```python
from build123d import *

# Parameters (mm, degrees)
BOSS_EXTRUDE2_DEPTH = 6.35
SKETCH5_R           = 1.778
CUT_EXTRUDE1_DEPTH  = 6.35
SKETCH7_W           = 6.35
SKETCH7_H           = 12.7
BOSS_EXTRUDE3_DEPTH = 6.35
SKETCH8_R           = 1.778
CUT_EXTRUDE3_DEPTH  = 6.35
SKETCH9_R           = 1.143
CUT_EXTRUDE4_DEPTH  = 12.7
BOSS_EXTRUDE5_DEPTH = 3.81
FILLET1_R           = 2.032
SKETCH12_R          = 1.143
CUT_EXTRUDE5_DEPTH  = 12.7


with BuildPart() as part:
    # Sketch2 → Boss-Extrude2 (new body)
    with BuildSketch(Plane.XY):
        Polygon((0, 0), (38.1, 0), (12.7, -43.994090512), (7.200738686, -40.819090512), (27.101477372, -6.35), (0, -6.35), align=None)
    extrude(amount=BOSS_EXTRUDE2_DEPTH)

    # Sketch5 → Cut-Extrude1 (cut)
    with BuildSketch(Plane(origin=(0, 0, 0), x_dir=(1, 0, 0), z_dir=(0, 1, 0))):
        with Locations((5.08, -3.175)):
            Circle(SKETCH5_R)
        with Locations((24.638, -3.175)):
            Circle(SKETCH5_R)
    extrude(amount=-CUT_EXTRUDE1_DEPTH, mode=Mode.SUBTRACT)

    # Sketch7 → Boss-Extrude3 (add)
    with BuildSketch(Plane(origin=(0, 0, 0), x_dir=(1, 0, 0), z_dir=(0, 1, 0))):
        with Locations((14.859, 6.35)):
            Rectangle(SKETCH7_W, SKETCH7_H)
    extrude(amount=-BOSS_EXTRUDE3_DEPTH)

    # Sketch8 → Cut-Extrude3 (cut)
    with BuildSketch(Plane(origin=(0, 0, 0), x_dir=(1, 0, 0), z_dir=(0, 1, 0))):
        with Locations((14.859, 6.604)):
            Circle(SKETCH8_R)
    extrude(amount=-CUT_EXTRUDE3_DEPTH, mode=Mode.SUBTRACT)

    # Sketch9 → Cut-Extrude4 (cut)
    with BuildSketch(Plane.XY.offset(6.35)):
        with Locations((11.537869343, -39.656959855)):
            Circle(SKETCH9_R)
        with Locations((25.537841343, -15.408297047)):
            Circle(SKETCH9_R)
    extrude(amount=-CUT_EXTRUDE4_DEPTH, mode=Mode.SUBTRACT)

    # Sketch11 → Boss-Extrude5 (add)
    with BuildSketch(Plane(origin=(0, 0, 0), x_dir=(-1, 0, 0), z_dir=(0, 0, -1))):
        Polygon((-29.874972, -14.24616639), (-24.375710686, -11.07116639), (-21.200710686, -16.570427704), (-26.699972, -19.745427704), align=None)
        Polygon((-15.875, -38.494829198), (-10.375738686, -35.319829198), (-7.200738686, -40.819090512), (-12.7, -43.994090512), align=None)
    extrude(amount=BOSS_EXTRUDE5_DEPTH)

    # Fillet1
    fillet1_edges = [part.edges().sort_by_distance(p)[0] for p in [
        (0, 0, 3.175),
        (38.1, 0, 3.175),
        (0, -6.35, 3.175),
        (11.684, -3.175, 0),
        (11.684, -3.175, -12.7),
        (18.034, -3.175, -12.7),
        (18.034, -3.175, 0),
    ]]
    fillet(fillet1_edges, radius=FILLET1_R)

    # Sketch12 → Cut-Extrude5 (cut)
    with BuildSketch(Plane.XY.offset(6.35)):
        with Locations((25.537841343, -15.408297047)):
            Circle(SKETCH12_R)
        with Locations((11.537869343, -39.656959855)):
            Circle(SKETCH12_R)
    extrude(amount=-CUT_EXTRUDE5_DEPTH, mode=Mode.SUBTRACT)


solid = part.part
```
Geometry: final body of the model. Coordinates: model frame, mm. A direction names the side the tool comes from. Give positions to 0.01 mm unless a question says otherwise; leave off trailing zeros. Write each loop counter-clockwise with the first axis right and the second up, starting at its lowest first coordinate (ties: lowest second). Pieces come first, ordered by that corner, then holes.
1. Section query D-D, the plane y = -32. Return loops of the section in (x, z).
2. Section query B-B, the plane z = -6. Return loops of the section in (x, y), then the cut area to 3 significant figures.
3. Section query C-C, the plane x = 15. Return loops of the section in (y, z).
4. Section query A-A, the plane x = 5.08. Return loops of the section in (y, z).
5. Pin query (flat end, axial travel): P1, Ø11.5, axis at x = 29.5, y = -4, coming from the -Z side; P2, Ø2.5, axis at x = 9.5, y = -41.5, coming from the -Z side; P3, Ø2, axis at x = 11.54, y = -39.66, coming from the +Z side; P4, Ø6, axis at y = -20.5, z = 0, coming from the +X side. Return the tip coordinate at first contact, or that it passes through.
6. Reachability of faces 4 (the flat face through (5, -3, 0)), 5 (the flat face through (27.2, -12.7, -1.9)), 6 (the flat face through (13.164, -36.93, -1.878)), 7 (the flat face through (12, -41, -3.81)) from +Z, -Z, +X, -X, +Y, -Y: full face, straight path, thin tool, end or side. Return the list, or none.
7. Draft query along Z for faces 1 (the cylindrical face through (26.334, -3.131, 2.641)), 2 (the cylindrical face through (36.325, -0.99, 3.219)), 3 (the cylindrical face through (12.263, -3.219, -12.089)). Return one class per face: released by +Z, released by -Z, zero draft, split by the parting line, or undercut.
8. Line query: probe 1 along Z at (x, y) = (5, -4); probe 2 along Z at (x, y) = (27, -15.5); probe 3 along X at (y, z) = (-15.5, 2.5). Output: solid intervals per line, ascending.
Computed:
1. outline: (12.29, 0) - (19.62, 0) - (19.62, 6.35) - (12.29, 6.35) - close
2. outline: (11.68, -6.35) - (13.19, -6.35) - (13.19, 0) - (11.68, 0) - close; (16.53, -6.35) - (18.03, -6.35) - (18.03, 0) - (16.53, 0) - close
2. area: 19.1 mm2
3. outline: (-40.01, -3.81) - (-37.99, -3.81) - (-37.99, 0) - (-27.31, 0) - (-27.31, 6.35) - (-40.01, 6.35) - close; (-6.35, -12.7) - (0, -12.7) - (0, -8.38) - (-6.35, -8.38) - close; (-6.35, -4.83) - (0, -4.83) - (0, 6.35) - (-6.35, 6.35) - close
4. outline: (-6.35, 0) - (0, 0) - (0, 1.4) - (-6.35, 1.4) - close; (-6.35, 4.95) - (0, 4.95) - (0, 6.35) - (-6.35, 6.35) - close
5. P1: stops at z = 0
5. P2: stops at z = -3.81
5. P3: passes through
5. P4: stops at x = 28
6. face 4: -Z, -X, +Y
6. face 5: -Z, +X, +Y
6. face 6: -Z, +X
6. face 7: -Z, +X, -X, -Y
7. face 1: undercut
7. face 2: zero draft
7. face 3: released by -Z
8. probe 1: z = 0 to 1.4, 4.95 to 6.35
8. probe 2: z = -3.81 to 6.35
8. probe 3: x = 21.82 to 24.4, 26.68 to 29.15
